Autodesk Fusion 360 part; units mm, degrees
sketch "Sketch1" plane through (0, 0, 0) normal (0, 0, 1) x (1, 0, 0) in component "ZSY Standoff"
  line L0 (0, 0) -> (20, 0)
  line L1 (20, 0) -> (20, 20)
  line L2 (20, 20) -> (0, 20)
  line L3 (0, 20) -> (0, 0)
  line L4 (0, 17.5) -> (20, 17.5) construction
  line L5 (10, 20) -> (10, 0) construction
  circle A0 centre (17.5, 17.5) radius 1.6
  circle A1 centre (2.5, 17.5) radius 1.6
  line L6 (2, 20) -> (2, 0) construction
  line L7 (18, 20) -> (18, 0) construction
  line L8 (0, 3) -> (20, 3) construction
  line L9 (0, 15) -> (20, 15) construction
  line L10 (2, 15) -> (18, 15)
  line L11 (18, 15) -> (18, 3)
  line L12 (18, 3) -> (2, 3)
  line L13 (2, 3) -> (2, 15)
  dimension "d1" = 20
  dimension "d2" = 20
  dimension "d3" = 2.5
  dimension "d4" = 3.2
  dimension "d5" = 3.2
  dimension "d6" = 7.5
  dimension "d7" = 7.5
  dimension "d8" = 2
  dimension "d9" = 2
  dimension "d10" = 3
  dimension "d11" = 5
extrude "Extrude1" add sketch "Sketch1" along normal blind 3 in component "ZSY Standoff"
fillet "Fillet1" radius 1.5 4 edges at (20, 20, 1.5) (0, 20, 1.5) (0, 0, 1.5) (20, 0, 1.5) in component "ZSY Standoff"
fillet "Fillet2" radius 1 4 edges at (2, 15, 1.5) (18, 15, 1.5) (18, 3, 1.5) (2, 3, 1.5) in component "ZSY Standoff"
component "ZSY Standoff" placed x (1, 0, 0) y (0, 1, 0) z (0, 0, 1) at (0, 0, 0)
Design review of the part built by this model. Coordinates are the model's own, in mm. A direction names the side the tool comes from. Give positions to 0.01 mm unless a question says otherwise; leave off trailing zeros. Write each loop counter-clockwise with the first axis right and the second up, starting at its lowest first coordinate (ties: lowest second). Pieces come first, ordered by that corner, then holes. Notation, with made-up numbers: M -12,78.25 L 23,78.25 A16 cw 23,105.25 Z; hole C 78,-9 d3. An arc over 180 degrees is marked long. Return JSON: item names as keys, results as strings. Group by question number.
Item 1: Take a section at D-D (x = 8.25). Give the boundary of the cut face in (y, z).
Item 2: Wall thickness on line 1 along Y through (x, z) = (6.25, 0.9); line 2 along Y through (x, z) = (17.5, 1.4); line 3 along X through (y, z) = (7, 2.25): over which ranges is each line inside the solid? List them lowest first.
Item 3: Tool access review of faces 1 (the flat face through (10, 20, 1)), 2 (the flat face through (10, 15, 1)): name each direction out of +Z, -Z, +X, -X, +Y, -Y from which nothing blocks a thin tool from reaching the whole face with its end or side.
Item 4: Take a section at C-C (y = 17.5). Give the boundary of the cut face in (x, z), plus the area to 3 significant figures.
Item 5: Take a section at B-B (z = 1.75). Give the boundary of the cut face in (x, y).
Item 6: Clearance check with flat-ended pins moving along their axes: pin 1 Ø3 at (x, y) = (17.5, 17.5) entering from -Z; pin 2 Ø6 at (x, y) = (4, 13) entering from -Z. State where each tip first meets the part, or that it passes through.
Item 7: Take a section at A-A (y = 8.25). Give the boundary of the cut face in (x, z).
Return value:
{
 "1": {"outline": "M 0,0 L 3,0 L 3,3 L 0,3 Z; M 15,0 L 20,0 L 20,3 L 15,3 Z"},
 "2": {"line 1": "y = 0 to 3, 15 to 20", "line 2": "y = 0 to 3.13, 14.87 to 15.9, 19.1 to 20", "line 3": "x = 0 to 2, 18 to 20"},
 "3": {"face 1": "+Z, -Z, +X, -X, +Y", "face 2": "+Z, -Z"},
 "4": {"outline": "M 0,0 L 0.9,0 L 0.9,3 L 0,3 Z; M 4.1,0 L 15.9,0 L 15.9,3 L 4.1,3 Z; M 19.1,0 L 20,0 L 20,3 L 19.1,3 Z", "area": "40.8 mm2"},
 "5": {"outline": "M 0,1.5 A1.5 ccw 1.5,0 L 18.5,0 A1.5 ccw 20,1.5 L 20,18.5 A1.5 ccw 18.5,20 L 1.5,20 A1.5 ccw 0,18.5 Z; hole C 2.5,17.5 d3.2; hole M 2,4 A1 ccw 3,3 L 17,3 A1 ccw 18,4 L 18,14 A1 ccw 17,15 L 3,15 A1 ccw 2,14 Z; hole C 17.5,17.5 d3.2"},
 "6": {"pin 1": "passes through", "pin 2": "stops at z = 0"},
 "7": {"outline": "M 0,0 L 2,0 L 2,3 L 0,3 Z; M 18,0 L 20,0 L 20,3 L 18,3 Z"}
}
